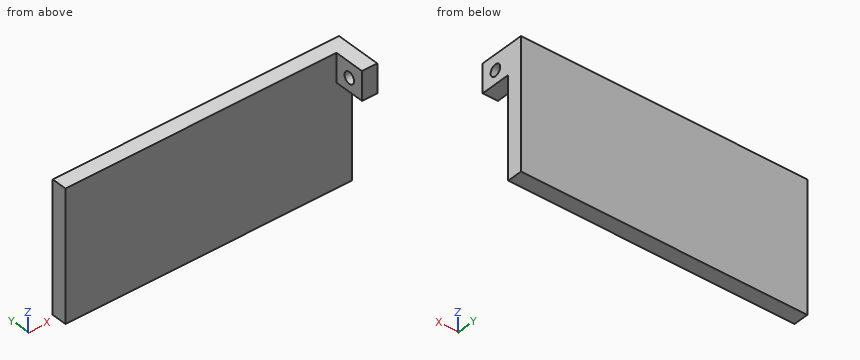
from build123d import *

# Parameters (mm, degrees)
F0_W     = 150
F0_H     = 68
F1_DEPTH = 8
F2_W     = 24
F2_H     = 15
F2_R     = 3
F3_DEPTH = 8


with BuildPart() as f1:
    # F0 (on Front) → F1 (new body)
    with BuildSketch(Plane.XZ):
        with Locations((-75, -34)):
            Rectangle(F0_W, F0_H)
    extrude(amount=F1_DEPTH)

    # F2 (on face) → F3 (join)
    with BuildSketch(Plane.YZ):
        with Locations((-12, -7.5)):
            Rectangle(F2_W, F2_H)
        with Locations((-16, -8)):
            Circle(F2_R, mode=Mode.SUBTRACT)
    extrude(amount=-F3_DEPTH)


solid = f1.part
Model file for the job. Use its own axes, mm. Round coordinates to 2 decimals unless told otherwise and drop trailing zeros. Loops run counter-clockwise (first coordinate to the right, second up) from the corner with the lowest first, then second, coordinate; pieces in that order, holes last. Notation, with made-up numbers: M -22.5,-17.5 L -11.5,-17.5 A10 cw -11.5,-11.5 Z; hole C -31.75,-9 d6. An arc over 180 degrees is marked long. One line per question, with ' | ' between items.
1) Band-saw the part on B-B (y = -16). Give the cut face in (x, z).
Solved:
outline: M -8,-15 L 0,-15 L 0,-11 L -8,-11 Z; M -8,-5 L 0,-5 L 0,0 L -8,0 Z
2) Band-saw the part on C-C (x = -72). Give the cut face in (y, z).
Solved:
outline: M -8,-68 L 0,-68 L 0,0 L -8,0 Z
3) Drill centre lines: line 1 along Z through (x, y) = (-3, -16); line 2 along Y through (x, z) = (-90, -36). Where is each one in solid material? Low to high.
Solved:
line 1: z = -15 to -11, -5 to 0 | line 2: y = -8 to 0
4) Band-saw the part on D-D (z = -46.5). Give the cut face in (x, y), then the cut area to 3 significant figures.
Solved:
outline: M -150,-8 L 0,-8 L 0,0 L -150,0 Z | area: 1,200 mm²
5) Flat gauge pins, fed straight in: pin 1 (4 mm diameter, centred on x = -5.5, y = -18, fed in from -Z); pin 2 (1.5 mm diameter, centred on x = -61, y = -10.5, fed in from -Z); pin 3 (6 mm diameter, centred on y = -20.5, z = -12, fed in from -X). Where does each tip first touch, or does it go through?
Solved:
pin 1: stops at z = -15 | pin 2: passes through | pin 3: stops at x = -8
6) Band-saw the part on A-A (z = -8). Give the cut face in (x, y), then the cut area to 3 significant figures.
Solved:
outline: M -150,-8 L -8,-8 L -8,-13 L 0,-13 L 0,0 L -150,0 Z; M -8,-24 L 0,-24 L 0,-19 L -8,-19 Z | area: 1,280 mm²
